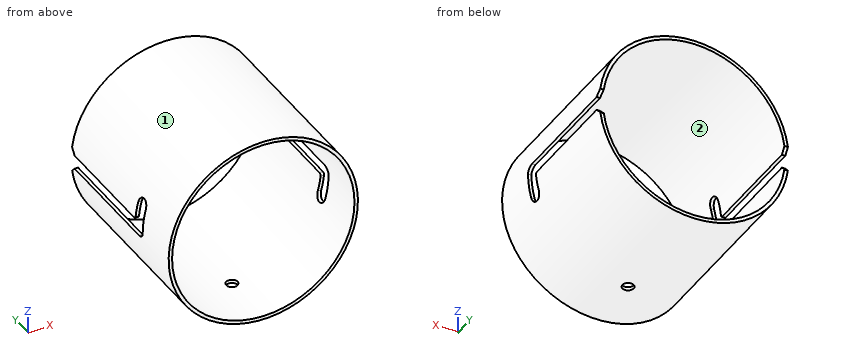
from build123d import *

# Parameters (mm, degrees)
SKETCH2_W                    = 3
SKETCH2_H                    = 155
CUT_EXTRUDE1_DEPTH           = 83.55
FILLET1_R                    = 6
CHAMFER1_SIZE                = 5
FILLET4_R                    = 2
CIRPATTERN1_COUNT            = 2
FILLET1_OF_CIRPATTERN1_R     = 6
CHAMFER1_OF_CIRPATTERN1_SIZE = 5
FILLET4_OF_CIRPATTERN1_R     = 2
SKETCH4_R                    = 5
CUT_EXTRUDE2_DEPTH           = 100


with BuildPart() as part:
    # Sketch2 → Revolve1 (revolve)
    with BuildSketch(Plane(origin=(0, 0, 0), x_dir=(0, 0, -1), z_dir=(1, 0, 0))):
        with Locations((-81.05, 77.5)):
            Rectangle(SKETCH2_W, SKETCH2_H)
    revolve(axis=Axis((0, -7.75, 0), (0, 1, 0)))

    # Sketch3 → Cut-Extrude1 (cut, through all)
    with BuildSketch(Plane(origin=(0, 0, 0), x_dir=(0, 0, -1), z_dir=(1, 0, 0))):
        with BuildLine():
            Line((-6, 155), (6, 155))
            Line((6, 155), (6, 41.3))
            Line((6, 41.3), (-21, 41.3))
            ThreePointArc((-21, 41.3), (-27, 47.3), (-21, 53.3))
            Line((-21, 53.3), (-6, 53.3))
            Line((-6, 53.3), (-6, 155))
        make_face()
    cut_extrude1 = extrude(amount=-CUT_EXTRUDE1_DEPTH, mode=Mode.SUBTRACT)

    # Fillet1
    fillet1_edges = [part.edges().sort_by_distance(p)[0] for p in [
        (-80.82753304, 41.3, -6),
    ]]
    fillet(fillet1_edges, radius=FILLET1_R)

    # Chamfer1
    chamfer1_edges = [part.edges().sort_by_distance(p)[0] for p in [
        (-80.82753304, 155, -6),
        (-80.82753304, 155, 6),
    ]]
    chamfer(chamfer1_edges, length=CHAMFER1_SIZE)

    # Fillet4
    fillet4_edges = [part.edges().sort_by_distance(p)[0] for p in [
        (-80.82753304, 53.3, 6),
    ]]
    fillet(fillet4_edges, radius=FILLET4_R)

    # CirPattern1: Cut-Extrude1 ×2 about axis
    cirpattern1_axis = Axis((0, -7.75, 0), (0, 1, 0))
    for i in range(1, CIRPATTERN1_COUNT):
        add(cut_extrude1.rotate(cirpattern1_axis, i * 360 / CIRPATTERN1_COUNT), mode=Mode.SUBTRACT)

    # Fillet1 of CirPattern1
    fillet1_of_cirpattern1_edges = [part.edges().sort_by_distance(p)[0] for p in [
        (80.82753304, 41.3, 6),
    ]]
    fillet(fillet1_of_cirpattern1_edges, radius=FILLET1_OF_CIRPATTERN1_R)

    # Chamfer1 of CirPattern1
    chamfer1_of_cirpattern1_edges = [part.edges().sort_by_distance(p)[0] for p in [
        (80.82753304, 155, 6),
        (80.82753304, 155, -6),
    ]]
    chamfer(chamfer1_of_cirpattern1_edges, length=CHAMFER1_OF_CIRPATTERN1_SIZE)

    # Fillet4 of CirPattern1
    fillet4_of_cirpattern1_edges = [part.edges().sort_by_distance(p)[0] for p in [
        (80.82753304, 53.3, -6),
    ]]
    fillet(fillet4_of_cirpattern1_edges, radius=FILLET4_OF_CIRPATTERN1_R)

    # Sketch4 → Cut-Extrude2 (cut)
    with BuildSketch(Plane.XY):
        with Locations((0, 50)):
            Circle(SKETCH4_R)
    extrude(amount=-CUT_EXTRUDE2_DEPTH, mode=Mode.SUBTRACT)


solid = part.part
Input: part model. Units: mm. Frame: model coordinates. Face numbers are marked on the shaded views. Give positions to 0.01 mm unless a question says otherwise; leave off trailing zeros. Write each loop counter-clockwise with the first axis right and the second up, starting at its lowest first coordinate (ties: lowest second). Pieces come first, ordered by that corner, then holes.
Q1. Section D-D, the plane y = 50. Output: boundary loops of the cut face in (x, z), plus the area to 3 significant figures.
Q2. First-contact query: P1, Ø1, axis at x = 41, y = 88, coming from the -Z side; P2, Ø6, axis at x = -9, y = 127.5, coming from the +Z side; P3, Ø1.6, axis at x = 79.5, z = -14, coming from the -Y side; P4, Ø12, axis at x = -64.5, y = 92.5, coming from the -Z side. Flat tips, straight axial feed; report the tip coordinate or a pass-through.
Q3. Pull-direction query (X, two-part tool) for the marked faces 1 and 2; classes: pulls with the +X half, pulls with the -X half, needs draft (parallel to the pull), parting line crosses it, or undercut.
Q4. Section B-B, the plane x = 0. Output: boundary loops of the cut face in (y, z), plus the area to 3 significant figures.
Q5. Section A-A, the plane y = 99. Output: boundary loops of the cut face in (x, z), plus the area to 3 significant figures.
Q6. Material intervals for probe 1 along Z at (x, y) = (-0.5, 99); probe 2 along Z at (x, y) = (30, 148.5), sorted ascending.
Q7. Section C-C, the plane z = 64.5. Output: boundary loops of the cut face in (x, y).
Filled in:
1. outline: (-82.33, -6) arc R82.55 ccw to (-5, -82.4) - (-5, -79.39) arc R79.55 cw to (-79.32, -6) - close; (-78.23, 26.36) - (-75.06, 26.36) arc R79.55 cw to (79.32, 6) - (82.33, 6) arc R82.55 ccw to start; (5, -82.4) arc R82.55 ccw to (78.23, -26.36) - (75.06, -26.36) arc R79.55 cw to (5, -79.39) - close
1. area: 1,300 mm2
2. P1: stops at z = -71.93
2. P2: stops at z = 82.33
2. P3: stops at y = 0
2. P4: stops at z = -58.24
3. face 1: parting line crosses it
3. face 2: undercut
4. outline: (0, -82.55) - (45, -82.55) - (45, -79.55) - (0, -79.55) - close; (0, 79.55) - (155, 79.55) - (155, 82.55) - (0, 82.55) - close; (55, -82.55) - (155, -82.55) - (155, -79.55) - (55, -79.55) - close
4. area: 900 mm2
5. outline: (-82.33, -6) arc R82.55 ccw to (82.33, -6) - (79.32, -6) arc R79.55 cw to (-79.32, -6) - close; (-82.33, 6) - (-79.32, 6) arc R79.55 cw to (79.32, 6) - (82.33, 6) arc R82.55 ccw to start
5. area: 1,460 mm2
6. probe 1: z = -82.55 to -79.55, 79.55 to 82.55
6. probe 2: z = -76.91 to -73.68, 73.68 to 76.91
7. outline: (-51.52, 0) - (-46.56, 0) - (-46.56, 155) - (-51.52, 155) - close; (46.56, 0) - (51.52, 0) - (51.52, 155) - (46.56, 155) - close
